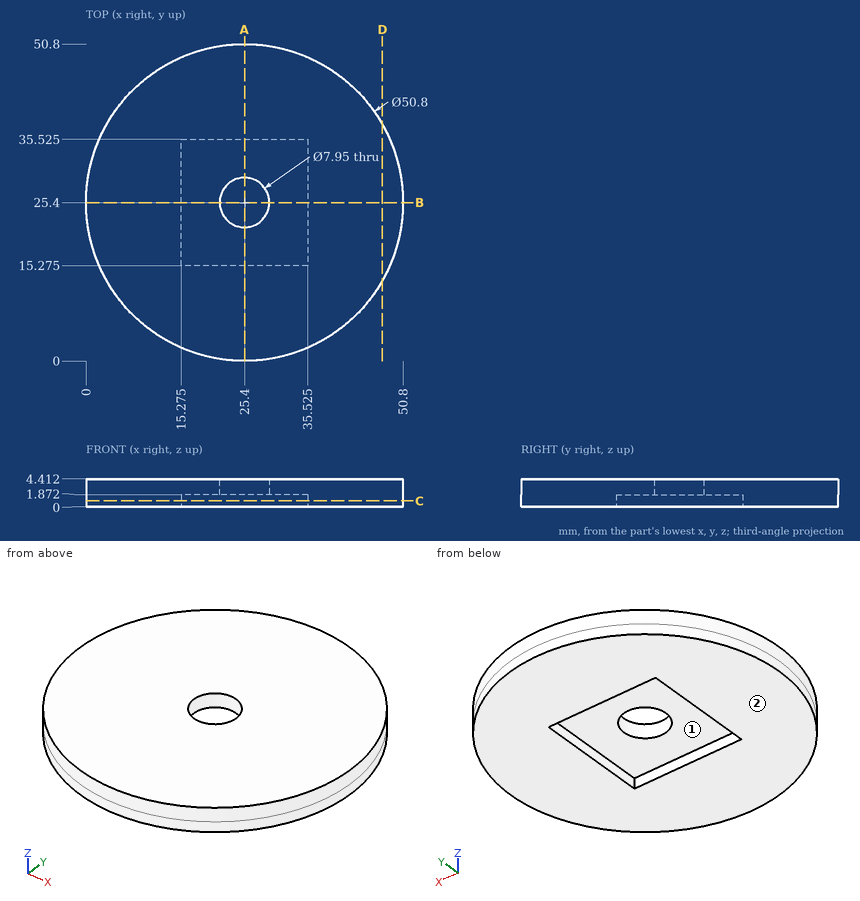
Here's the drawing with two shaded views (mm, measured from the low corner). I have some questions. Round coordinates to 2 decimals unless told otherwise and drop trailing zeros. Loops run counter-clockwise (first coordinate to the right, second up) from the corner with the lowest first, then second, coordinate; pieces in that order, holes last. Notation, with made-up numbers: (-3.75, 45) - (26.25, 45) arc R37 ccw to (26.25, 84) - close; hole circle Ø5 at (50, 44.5). An arc over 180 degrees is marked (long way). Write item = value, one per line.
1) If we mould it in two halves opening along X, with no side actions, what happens to the marked faces 1 and 2? For each: pulls with the +X half, pulls with the -X half, needs draft (parallel to the pull), parting line crosses it, or undercut.
Computed:
face_1 = undercut
face_2 = needs draft
2) Imagine slicing it at C-C (z = 0.9). Please give me the cut outline in (x, y) (1 decimal), and give its area (3 significant figures).
Computed:
outline = circle Ø50.8 at (25.4, 25.4); hole (15.3, 15.3) - (35.5, 15.3) - (35.5, 35.5) - (15.3, 35.5) - close
area = 1,620 mm2
3) I need wall thicknesses on line 1 along Y through (x, z) = (25.4, 3.7) (1 decimal); line 2 along Y through (x, z) = (26, 3); line 3 along Z through (x, y) = (18, 30.5). Which ranges of each line are inside material? Lowest first, please. Write a range as from..to.
Computed:
line_1 = 0..21.4, 29.4..50.8
line_2 = 0.01..21.47, 29.33..50.79
line_3 = 1.87..4.41
4) I'm going to push flat-ended pins straight in: P1, Ø2, axis at x = 22.5, z = 1, coming from the -Y side; P2, Ø1.5, axis at y = 24.5, z = 1, coming from the +X side; P3, Ø0.9, axis at x = 22.5, z = 1, coming from the +Y side. Where does each tip first touch, or does it pass through?
Computed:
P1 = 0.07
P2 = 50.8
P3 = 50.68
5) Imagine slicing it at D-D (x = 47.5). Please give me the cut outline in (y, z).
Computed:
outline = (12.88, 0) - (37.92, 0) - (37.92, 4.41) - (12.88, 4.41) - close
6) Imagine slicing it at A-A (x = 25.4). Please give me the cut outline in (y, z) (1 decimal), and give its area (3 significant figures).
Computed:
outline = (0, 0) - (15.3, 0) - (15.3, 1.9) - (21.4, 1.9) - (21.4, 4.4) - (0, 4.4) - close; (29.4, 1.9) - (35.5, 1.9) - (35.5, 0) - (50.8, 0) - (50.8, 4.4) - (29.4, 4.4) - close
area = 166 mm2
